from build123d import *

# Parameters (mm, degrees)
F1_DEPTH = 25.4
F2_DEPTH = 4.572


with BuildPart() as f1:
    # F0 (on Front) → F1 (new body)
    with BuildSketch(Plane.XZ):
        with BuildLine():
            ThreePointArc((-7.3314444091, 37.387964947), (-24.2103486965, -29.4188547703), (38.1, 0))
            ThreePointArc((38.1, 0), (29.6258643924, 23.956589052), (7.9730625194, 37.2564125227))
            ThreePointArc((7.9730625194, 37.2564125227), (0.3274827628, 38.0985925598), (-7.3314444091, 37.387964947))
        make_face()
        with BuildLine():
            ThreePointArc((21.4790297282, -15.1774131634), (0, -36.6564428916), (-21.4790297282, -15.1774131634))
            Line((-21.4790297282, -15.1774131634), (21.4790297282, -15.1774131634))
        make_face(mode=Mode.SUBTRACT)
        Polygon((-6.5538821451, 0), (0, 10.348235436), (6.5538832613, 0), align=None, mode=Mode.SUBTRACT)
        Polygon((-16.5571787067, 6.5538827032), (-21.7312953085, 24.1458841722), (-9.3134132318, 20.3515308814), align=None, mode=Mode.SUBTRACT)
        Polygon((15.9893649439, 6.9261599984), (11.3830587563, 21.0414130949), (22.7661197451, 23.8009441816), align=None, mode=Mode.SUBTRACT)
    extrude(amount=F1_DEPTH)

    # F0 (on Front) → F2 (join)
    with BuildSketch(Plane.XZ):
        with BuildLine():
            ThreePointArc((-7.3314444091, 37.387964947), (0.3274827628, 38.0985925598), (7.9730625194, 37.2564125227))
            add(Edge.make_bspline(
                [(13.7976465038, 46.2221194713), (11.4257742807, 46.6512124753), (7.1192413466, 47.4336244295), (5.0852564917, 42.1322478947), (6.9696530621, 38.9708554427), (7.9730625194, 37.2564125227)],
                knots=[0, 0, 0, 0, 0.361306556, 0.6573311923, 1, 1, 1, 1], degree=3))
            Line((13.7976465038, 46.2221194713), (17.9369442501, 51.0512971987))
            add(Edge.make_bspline(
                [(-3.1044713563, 43.1176461616), (0.7883330685, 48.011810346), (7.7265818936, 56.7348092941), (14.8223562753, 52.7850063276), (17.9369442501, 51.0512971987)],
                knots=[0, 0, 0, 0, 0.5610644015, 1, 1, 1, 1], degree=3))
            add(Edge.make_bspline(
                [(-3.1044713563, 43.1176461616), (-4.5159470278, 41.2204233442), (-5.9199687377, 39.2851877643), (-7.3314444091, 37.387964947)],
                knots=[0, 0, 0, 0, 7.1201508418, 7.1201508418, 7.1201508418, 7.1201508418], degree=3))
        make_face()
    extrude(amount=F2_DEPTH)


solid = f1.part
Here's how the part is built. I have some questions about the finished solid (model axes, mm). A direction names the side the tool comes from. Round coordinates to 2 decimals unless told otherwise and drop trailing zeros. Order: outer loops, then holes, each group sorted by start corner. A loop starts at its lowest first (then second) coordinate and runs counter-clockwise, first axis right, second up. Notation, with made-up numbers: M -12,-21 L 7,-21 A13 cw 7,-11 Z; hole C 57,17.25 d1. An arc over 180 degrees is marked long. Return JSON: item names as keys, results as strings. Group by question number.
1. If we section it at B-B on y = -17.25: List the corners of the cut face in (x, z) for me, then the cut area to 3 significant figures.
2. Please list where these lines run through material, in increasing order: probe 1 along X at (y, z) = (-17.75, 7.5); probe 2 along X at (y, z) = (-18, 9.5); probe 3 along X at (y, z) = (-1.25, 12).
3. I'm going to push flat-ended pins straight in: pin 1 Ø5 at (x, z) = (6.5, 25) entering from +Y; pin 2 Ø12.5 at (x, y) = (-2, -11.5) entering from -Z; pin 3 Ø5 at (x, y) = (19.5, -22) entering from -Z; pin 4 Ø8.5 at (x, z) = (7.5, 42) entering from -Y. Where does each tip first touch, or does it pass through?
4. If we section it at D-D on x = 31.5: List the corners of the cut face in (y, z) for me.
5. If we mould it in two halves opening along Z, with no side actions, what happens to faces 1 (the face through (8, -25.4, 1)), 2 (the face through (-15.609, -12.522, 22.275))? For each: pulls with the +Z half, pulls with the -Z half, needs draft (parallel to the pull), parting line crosses it, or undercut.
6. If we section it at A-A on z = 22.5: List the corners of the cut face in (x, y) for me, then the cut area to 3 significant figures.
7. If we section it at C-C on x = 20: List the corners of the cut face in (y, z) for me.
8. On a 3-axis mill with a long thin cutter (end or side, diameter ignored), from which of +Z, -Z, +X, -X, +Y, -Y can I reach the whole of each face in a straight line? I mean faces 3 (the face through (-1, 0, 10)), 4 (the face through (0, -13, -15.177)), 5 (the face through (15.838, -2.254, 48.603)). Say none if no direction works.
Reply:
{
 "1": {"outline": "C 0,0 d76.2; hole M -21.73,24.15 L -16.56,6.55 L -9.31,20.35 Z; hole M -21.48,-15.18 A21.48 ccw 21.48,-15.18 Z; hole M -6.55,0 L 6.55,0 L 0,10.35 Z; hole M 11.38,21.04 L 15.99,6.93 L 22.77,23.8 Z", "area": "3,580 mm^2"},
 "2": {"probe 1": "-37.35 to -16.84, -16.06 to -1.8, 1.8 to 15.8, 16.22 to 37.35", "probe 2": "-36.9 to -17.42, -15.01 to -0.54, 0.54 to 15.15, 17.02 to 36.9", "probe 3": "-36.16 to -18.16, -13.7 to 14.33, 18.03 to 36.16"},
 "3": {"pin 1": "y = 0", "pin 2": "z = -38.1", "pin 3": "z = -34.1", "pin 4": "y = -4.57"},
 "4": {"outline": "M -25.4,-21.43 L 0,-21.43 L 0,21.43 L -25.4,21.43 Z"},
 "5": {"face 1": "needs draft", "face 2": "undercut"},
 "6": {"outline": "M -30.75,-25.4 L -21.25,-25.4 L -21.25,0 L -30.75,0 Z; M -16.34,-25.4 L 17.4,-25.4 L 17.4,0 L -16.34,0 Z; M 22.24,-25.4 L 30.75,-25.4 L 30.75,0 L 22.24,0 Z", "area": "1,310 mm^2"},
 "7": {"outline": "M -25.4,-32.43 L 0,-32.43 L 0,-23.01 L -25.4,-23.01 Z; M -25.4,-15.18 L 0,-15.18 L 0,16.91 L -25.4,16.91 Z; M -25.4,23.13 L 0,23.13 L 0,32.43 L -25.4,32.43 Z"},
 "8": {"face 3": "+Z, -Z, +X, -X, +Y", "face 4": "+Y, -Y", "face 5": "+X, +Y, -Y"}
}
